Geometry: see drawing. Coordinates: mm, zero at the bounding-box minimum. A direction names the side the tool comes from. Give positions to 0.01 mm unless a question says otherwise; leave off trailing zeros. Write each loop counter-clockwise with the first axis right and the second up, starting at its lowest first coordinate (ties: lowest second). Pieces come first, ordered by that corner, then holes. Notation, with made-up numbers: M 51.5,11.5 L 89.5,11.5 A14 ccw 89.5,23.5 Z; hole C -12.75,-4 d1. An arc over 180 degrees is marked long. Use a Markdown table: item, result. Add a question column.
(1) Draft query along X for the marked faces 1, 2 and 3. Return one class per face: released by +X, released by -X, zero draft, split by the parting line, or undercut.
(2) Material intervals for L1, parallel to Z at x = 9, y = 2; L2, parallel to X at y = 5.5, z = 8 (1 decimal); L3, parallel to X at y = 7.5, z = 8.25, sorted ascending.
(3) Reachability of the marked faces 4, 5 and 6 from +Z, -Z, +X, -X, +Y, -Y: full face, straight path, thin tool, end or side. Return the list, or none.
(4) Cut plane B-B (x = 10.25). Output: boundary loops of the cut face in (y, z).
(5) Pin query (flat end, axial travel): pin 1 Ø2 at (x, z) = (6.5, 26) entering from -Y; pin 2 Ø5 at (y, z) = (10.5, 3.5) entering from -X; pin 3 Ø3 at (y, z) = (5, 8.5) entering from +X. Return the tip coordinate at first contact, or that it passes through.
(6) Cut plane A-A (y = 7.75). Output: boundary loops of the cut face in (x, z) (1 decimal).
(7) Cut plane D-D (z = 4). Output: boundary loops of the cut face in (x, y) (1 decimal).
(8) Cut plane C-C (y = 4). Output: boundary loops of the cut face in (x, z), plus the area to 3 significant figures.
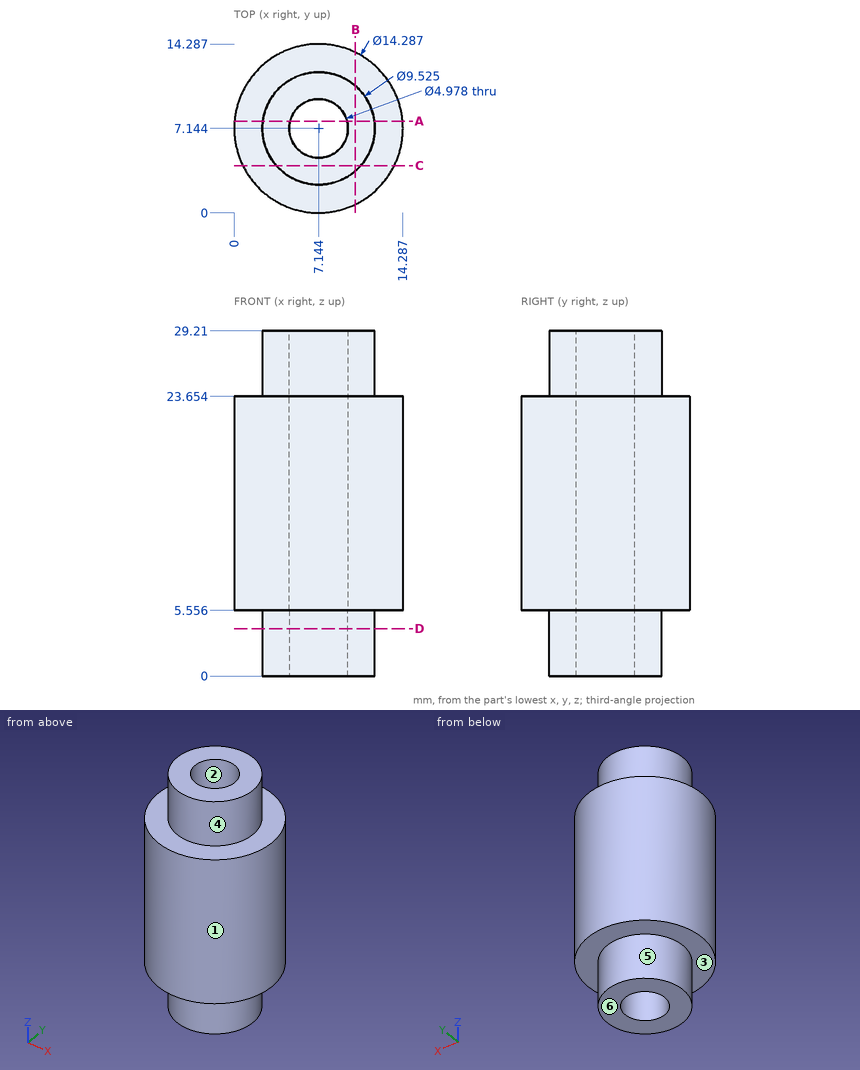
Answer list:
| question | item | result |
|---|---|---|
| 1 | face 1 | split by the parting line |
| 1 | face 2 | undercut |
| 1 | face 3 | zero draft |
| 2 | L1 | 5.56 to 23.65 |
| 2 | L2 | 0.2 to 5.3, 9 to 14.1 |
| 2 | L3 | 0.01 to 4.68, 9.61 to 14.28 |
| 3 | face 4 | +Z |
| 3 | face 5 | -Z |
| 3 | face 6 | -Z, +X, -X, +Y, -Y |
| 4 | outline | M 0.71,5.56 L 3.53,5.56 L 3.53,0 L 10.75,0 L 10.75,5.56 L 13.58,5.56 L 13.58,23.65 L 10.75,23.65 L 10.75,29.21 L 3.53,29.21 L 3.53,23.65 L 0.71,23.65 Z |
| 5 | pin 1 | y = 2.38 |
| 5 | pin 2 | x = 0.27 |
| 5 | pin 3 | x = 14.26 |
| 6 | outline | M 0,5.6 L 2.4,5.6 L 2.4,0 L 4.7,0 L 4.7,29.2 L 2.4,29.2 L 2.4,23.7 L 0,23.7 Z; M 9.6,0 L 11.9,0 L 11.9,5.6 L 14.3,5.6 L 14.3,23.7 L 11.9,23.7 L 11.9,29.2 L 9.6,29.2 Z |
| 7 | outline | C 7.1,7.1 d9.5; hole C 7.1,7.1 d5 |
| 8 | outline | M 0.73,5.56 L 3.57,5.56 L 3.57,0 L 10.72,0 L 10.72,5.56 L 13.56,5.56 L 13.56,23.65 L 10.72,23.65 L 10.72,29.21 L 3.57,29.21 L 3.57,23.65 L 0.73,23.65 Z |
| 8 | area | 312 mm² |
